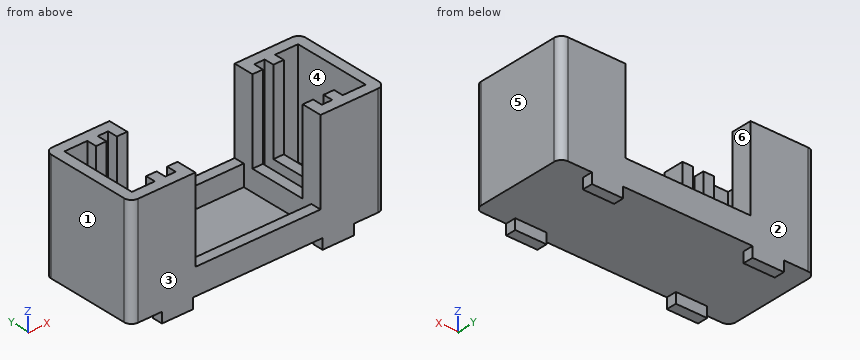
from build123d import *

# Parameters (mm, degrees)
SKETCH_W        = 24.4
SKETCH_H        = 9.4
PAD_DEPTH       = 10.5
SKETCH001_W     = 2.2
SKETCH001_H     = 7.4
SKETCH001_W_2   = 12
SKETCH001_W_3   = 1
POCKET_DEPTH    = 10
POCKET001_DEPTH = 8
SKETCH003_W     = 3
SKETCH003_H     = 1
PAD001_DEPTH    = 1
FILLET_R        = 0.7


with BuildPart() as part:
    # Sketch → Pad (new body)
    with BuildSketch(Plane.XY):
        with Locations((12.2, 4.7)):
            Rectangle(SKETCH_W, SKETCH_H)
    extrude(amount=PAD_DEPTH)

    # Sketch001 (on Face6 of Pad) → Pocket (cut)
    with BuildSketch(Plane.XY.offset(10.5)):
        with Locations((22.3, 4.7)):
            Rectangle(SKETCH001_W, SKETCH001_H)
        with Locations((2.1, 4.7)):
            Rectangle(SKETCH001_W, SKETCH001_H)
        with Locations((12.2, 4.7)):
            Rectangle(SKETCH001_W_2, SKETCH001_H)
        with Locations((4.7, 4.7)):
            Rectangle(SKETCH001_W_3, SKETCH001_H)
        with Locations((19.7, 4.7)):
            Rectangle(SKETCH001_W_3, SKETCH001_H)
    extrude(amount=-POCKET_DEPTH, mode=Mode.SUBTRACT)

    # Sketch002 (on Face5 of Pocket) → Pocket001 (cut)
    with BuildSketch(Plane.XY.offset(10.5)):
        Polygon((6.2, 9.4), (18.2, 9.4), (18.2, 7.45), (22.2, 7.45), (22.2, 1.95), (18.2, 1.95), (18.2, 0), (6.2, 0), (6.2, 1.95), (2.2, 1.95), (2.2, 7.45), (6.2, 7.45), align=None)
    extrude(amount=-POCKET001_DEPTH, mode=Mode.SUBTRACT)

    # Sketch003 (on Face2 of Pocket001) → Pad001 (join)
    with BuildSketch(Plane(origin=(0, 0, 0), x_dir=(1, 0, 0), z_dir=(0, 0, -1))):
        with Locations((4.5, -0.5)):
            Rectangle(SKETCH003_W, SKETCH003_H)
        with Locations((19.9, -0.5)):
            Rectangle(SKETCH003_W, SKETCH003_H)
        with Locations((4.5, -8.9)):
            Rectangle(SKETCH003_W, SKETCH003_H)
        with Locations((19.9, -8.9)):
            Rectangle(SKETCH003_W, SKETCH003_H)
    extrude(amount=PAD001_DEPTH)

    # Fillet
    fillet_edges = [part.edges().sort_by_distance(p)[0] for p in [
        (24.4, 0, 5.25),
        (0, 0, 5.25),
        (24.4, 9.4, 5.25),
        (0, 9.4, 5.25),
    ]]
    fillet(fillet_edges, radius=FILLET_R)


solid = part.part
Read the model definition and answer for the solid it produces. Units are mm, in the model's axes. Face numbers are marked on the shaded views. A direction names the side the tool comes from. Round coordinates to 2 decimals unless told otherwise and drop trailing zeros. Order: outer loops, then holes, each group sorted by start corner. A loop starts at its lowest first (then second) coordinate and runs counter-clockwise, first axis right, second up. Notation, with made-up numbers: (29.5, 7) - (88.5, 7) arc R19 cw to (88.5, 40) - close; hole circle Ø7 at (7, 18). An arc over 180 degrees is marked (long way). Use one line per item in the form item = value. Start each with the question number.
(1) The part is cut by section B-B (x = 5.5). Give the vertices of the cut face in (y, z), then the cut area to 3 significant figures.
(2) The part is cut by section D-D (z = 1.5). Give the vertices of the cut face in (x, y), then the cut area to 3 significant figures.
(3) The part is cut by section C-C (y = 3). Give the vertices of the cut face in (x, z).
(4) For the marked faces 5 and 6, determine the directions among +Z, -Z, +X, -X, +Y, -Y from which every point of the face is accessible in a straight line to the end or side of a thin tool.
(5) Determine the mould class of the marked faces 1, 2, 3 and 4 for opening direction Y: +Y half, -Y half, draft (parallel to the pull), parting line (faces both ways), or undercut.
(6) Find the intervals of material crossed by line 1 along X through (y, z) = (1.75, 6.75); line 2 along X through (y, z) = (8.5, 5.75); line 3 along Y through (x, z) = (16.25, 0.75), in increasing order. Write a range as from..to.
(7) The part is cut by section A-A (z = -0.5). Give the vertices of the cut face in (x, y).
(8) Flat-ended cylindrical pins translate along their axes: pin 1 Ø4 at (x, y) = (9, 2) entering from -Z; pin 2 Ø1.5 at (x, z) = (15.5, 4.5) entering from +Y; pin 3 Ø3 at (x, y) = (13, 6.5) entering from +Z. Find the tip coordinate at first contact, or state that the pin passes through.
Checked values:
q1.outline = (0, -1) - (1, -1) - (1, 0) - (8.4, 0) - (8.4, -1) - (9.4, -1) - (9.4, 10.5) - (7.45, 10.5) - (7.45, 2.5) - (1.95, 2.5) - (1.95, 10.5) - (0, 10.5) - close
q1.area = 56.7 mm^2
q2.outline = (0, 0.7) arc R0.7 ccw to (0.7, 0) - (23.7, 0) arc R0.7 ccw to (24.4, 0.7) - (24.4, 8.7) arc R0.7 ccw to (23.7, 9.4) - (0.7, 9.4) arc R0.7 ccw to (0, 8.7) - close; hole (1, 1) - (3.2, 1) - (3.2, 8.4) - (1, 8.4) - close; hole (4.2, 1) - (5.2, 1) - (5.2, 8.4) - (4.2, 8.4) - close; hole (6.2, 1) - (18.2, 1) - (18.2, 8.4) - (6.2, 8.4) - close; hole (19.2, 1) - (20.2, 1) - (20.2, 8.4) - (19.2, 8.4) - close; hole (21.2, 1) - (23.4, 1) - (23.4, 8.4) - (21.2, 8.4) - close
q2.area = 92.8 mm^2
q3.outline = (0, 0) - (24.4, 0) - (24.4, 10.5) - (23.4, 10.5) - (23.4, 0.5) - (21.2, 0.5) - (21.2, 2.5) - (20.2, 2.5) - (20.2, 0.5) - (19.2, 0.5) - (19.2, 2.5) - (18.2, 2.5) - (18.2, 0.5) - (6.2, 0.5) - (6.2, 2.5) - (5.2, 2.5) - (5.2, 0.5) - (4.2, 0.5) - (4.2, 2.5) - (3.2, 2.5) - (3.2, 0.5) - (1, 0.5) - (1, 10.5) - (0, 10.5) - close
q4.face_5 = +Z, -Z, +X, +Y, -Y
q4.face_6 = +Z
q5.face_1 = draft
q5.face_2 = +Y half
q5.face_3 = -Y half
q5.face_4 = undercut
q6.line_1 = 0..1, 3.2..4.2, 5.2..6.2, 18.2..19.2, 20.2..21.2, 23.4..24.4
q6.line_2 = 0..6.2, 18.2..24.4
q6.line_3 = 0..1, 8.4..9.4
q7.outline = (3, 0) - (6, 0) - (6, 1) - (3, 1) - close; (3, 8.4) - (6, 8.4) - (6, 9.4) - (3, 9.4) - close; (18.4, 0) - (21.4, 0) - (21.4, 1) - (18.4, 1) - close; (18.4, 8.4) - (21.4, 8.4) - (21.4, 9.4) - (18.4, 9.4) - close
q8.pin_1 = 0
q8.pin_2 = through
q8.pin_3 = 0.5
